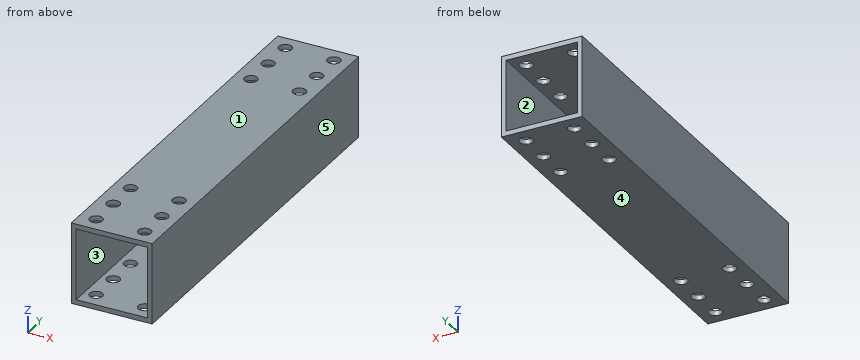
```python
from build123d import *

# Parameters (mm, degrees)
BOSS_EXTRUDE1_DEPTH      = 60
BOSS_EXTRUDE1_DEPTH_BACK = 60
SKETCH1_W                = 25
SKETCH1_H                = 25
SKETCH1_W_2              = 22
SKETCH1_H_2              = 22
SKETCH2_R                = 2
CUT_EXTRUDE1_DEPTH       = 25


with BuildPart() as part:
    # Sketch1 → Boss-Extrude1 (new, two sides: drawn at the far end of the back side and taken through both)
    with BuildSketch(Plane(origin=(0, 0, 0), x_dir=(1, 0, 0), z_dir=(0, 1, 0)).offset(-BOSS_EXTRUDE1_DEPTH_BACK)):
        Rectangle(SKETCH1_W, SKETCH1_H)
        Rectangle(SKETCH1_W_2, SKETCH1_H_2, mode=Mode.SUBTRACT)
    extrude(amount=BOSS_EXTRUDE1_DEPTH + BOSS_EXTRUDE1_DEPTH_BACK)

    # Sketch2 → Cut-Extrude1 (cut)
    with BuildSketch(Plane(origin=(0, 0, -12.5), x_dir=(-1, 0, 0), z_dir=(0, 0, -1))):
        with Locations((7.5, 55)):
            Circle(SKETCH2_R)
        with Locations((7.5, 45)):
            Circle(SKETCH2_R)
        with Locations((-7.5, 55)):
            Circle(SKETCH2_R)
        with Locations((-7.5, 45)):
            Circle(SKETCH2_R)
        with Locations((7.5, 35)):
            Circle(SKETCH2_R)
        with Locations((-7.5, 35)):
            Circle(SKETCH2_R)
    cut_extrude1 = extrude(amount=-CUT_EXTRUDE1_DEPTH, mode=Mode.SUBTRACT)

    # Mirror1: Cut-Extrude1 across plane
    add(cut_extrude1.mirror(Plane.ZX), mode=Mode.SUBTRACT)


solid = part.part
```
Can you work these out from the model? Positions are in its coordinate system, mm. Face numbers are marked on the shaded views. A direction names the side the tool comes from. Give positions to 0.01 mm unless a question says otherwise; leave off trailing zeros. Loops run counter-clockwise (first coordinate to the right, second up) from the corner with the lowest first, then second, coordinate; pieces in that order, holes last. Notation, with made-up numbers: M -28,23.25 L -15,23.25 A17 ccw -15,32.25 Z; hole C 46.25,45 d7. An arc over 180 degrees is marked long. Answer in a Markdown table with one row per item.
1. Which directions (+Z, -Z, +X, -X, +Y, -Y) give clear straight access to the entire face, cutting with the end or side of a thin tool? Please do the marked faces 1 and 2.
Taken from the geometry:
| item | result |
|---|---|
| face 1 | +Z, +X, -X, +Y, -Y |
| face 2 | +Y, -Y |
2. Thinking about a two-plate mould opening in X: for the marked faces 3, 4 and 5, which applies, released by +X, released by -X, zero draft, split by the parting line, or undercut?
Taken from the geometry:
| item | result |
|---|---|
| face 3 | undercut |
| face 4 | zero draft |
| face 5 | released by +X |
3. Suppose I cut it at A-A on z = -3.25. Write out the boundary of the cut face in (x, y), plus the area to 3 significant figures.
Taken from the geometry:
| item | result |
|---|---|
| outline | M -12.5,-60 L -11,-60 L -11,60 L -12.5,60 Z; M 11,-60 L 12.5,-60 L 12.5,60 L 11,60 Z |
| area | 360 mm² |
4. Suppose I cut it at B-B on y = -45. Write out the boundary of the cut face in (x, z), plus the area to 3 significant figures.
Taken from the geometry:
| item | result |
|---|---|
| outline | M -12.5,-12.5 L -9.5,-12.5 L -9.5,-11 L -11,-11 L -11,11 L -9.5,11 L -9.5,12.5 L -12.5,12.5 Z; M -5.5,-12.5 L 5.5,-12.5 L 5.5,-11 L -5.5,-11 Z; M -5.5,11 L 5.5,11 L 5.5,12.5 L -5.5,12.5 Z; M 9.5,-12.5 L 12.5,-12.5 L 12.5,12.5 L 9.5,12.5 L 9.5,11 L 11,11 L 11,-11 L 9.5,-11 Z |
| area | 117 mm² |
5. Suppose I cut it at C-C on x = -7.5. Count the separate pieces of the cut face and the enclosed holes in it, plus the area to 3 significant figures.
Taken from the geometry:
| item | result |
|---|---|
| separate pieces | 14 |
| enclosed holes | 0 |
| area | 288 mm² |
6. If I drill on line 1 along X through (y, z) = (-35, -11.5); line 2 along X through (y, z) = (-40.5, 3.5), over which ranges is the centre line in solid material (lowest first)?
Taken from the geometry:
| item | result |
|---|---|
| line 1 | x = -12.5 to -9.5, -5.5 to 5.5, 9.5 to 12.5 |
| line 2 | x = -12.5 to -11, 11 to 12.5 |
